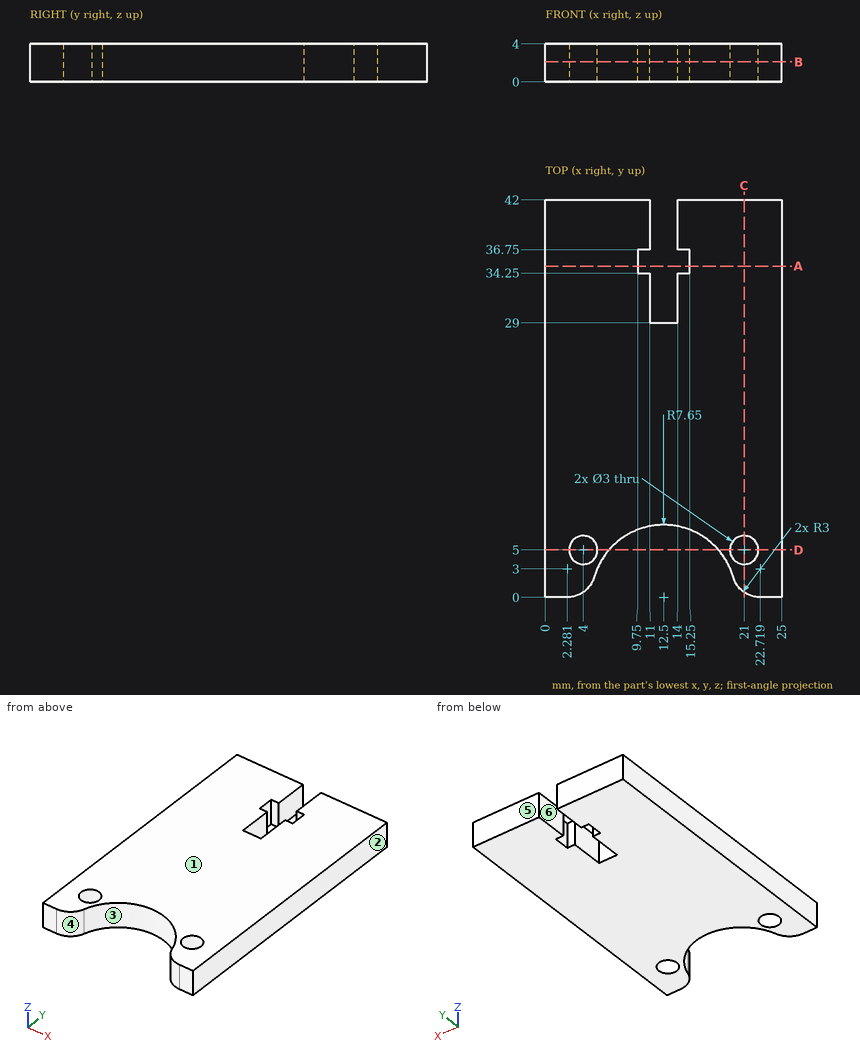
Could you check a few things on this drawing? It's one solid part, dimensions in mm from its lowest x, y, z. A direction names the side the tool comes from. Coordinates: 2 decimals unless noted, no trailing zeros. Order: outer loops, then holes, each group sorted by start corner. A loop starts at its lowest first (then second) coordinate and runs counter-clockwise, first axis right, second up. Notation, with made-up numbers: M 48.25,-21 L 57.25,-21 A23 ccw 57.25,1 Z; hole C -3.5,54 d8. An arc over 180 degrees is marked long. Use a Markdown table: item, result. Add a question column.
Q1. I want a section at A-A on y = 35. List the corners of the cut face in (x, z) for me, then the cut area to 3 significant figures.
Q2. I'm going to push flat-ended pins straight in: pin 1 (1.4 mm diameter, centred on x = 10, z = 2.5, fed in from -Y); pin 2 (1.5 mm diameter, centred on x = 12.5, z = 3, fed in from +Y); pin 3 (1.4 mm diameter, centred on x = 14.5, z = 1.5, fed in from -Y). Where does each tip first touch, or does it pass through?
Q3. We'd pull the mould along X, two halves only. Please class the marked faces 1, 2 and 3: pulls with the +X half, pulls with the -X half, needs draft (parallel to the pull), parting line crosses it, or undercut.
Q4. If I drill on L1, parallel to X at y = 4.5, z = 1.5 (1 decimal); L2, parallel to X at y = 6, z = 0.5 (1 decimal); L3, parallel to X at y = 38, z = 3.75, over which ranges is the centre line in solid material (lowest first)?
Q5. I want a section at B-B on z = 2.1. Give the number of separate pieces and of enclosed holes in the cut face, then the cut area to 3 significant figures.
Q6. Which directions (+Z, -Z, +X, -X, +Y, -Y) give clear straight access to the entire face, cutting with the end or side of a thin tool? Please do the marked faces 4, 5 and 6.
Q7. I want a section at C-C on x = 21. List the corners of the cut face in (y, z) for me.
Q8. I want a section at D-D on y = 5. List the corners of the cut face in (x, z) for me.
Checked values:
| question | item | result |
|---|---|---|
| 1 | outline | M 0,0 L 9.75,0 L 9.75,4 L 0,4 Z; M 15.25,0 L 25,0 L 25,4 L 15.25,4 Z |
| 1 | area | 78.0 mm² |
| 2 | pin 1 | y = 6.95 |
| 2 | pin 2 | y = 29 |
| 2 | pin 3 | y = 7.16 |
| 3 | face 1 | needs draft |
| 3 | face 2 | pulls with the +X half |
| 3 | face 3 | undercut |
| 4 | L1 | 0 to 2.6, 5.4 to 6.3, 18.7 to 19.6, 22.4 to 25 |
| 4 | L2 | 0 to 2.9, 5.1 to 7.8, 17.2 to 19.9, 22.1 to 25 |
| 4 | L3 | 0 to 11, 14 to 25 |
| 5 | separate pieces | 1 |
| 5 | enclosed holes | 2 |
| 5 | area | 896 mm² |
| 6 | face 4 | +Z, -Z, -Y |
| 6 | face 5 | +Z, -Z, +X, -X, +Y |
| 6 | face 6 | +Z, -Z, +Y |
| 7 | outline | M 0.54,0 L 3.5,0 L 3.5,4 L 0.54,4 Z; M 6.5,0 L 42,0 L 42,4 L 6.5,4 Z |
| 8 | outline | M 0,0 L 2.5,0 L 2.5,4 L 0,4 Z; M 5.5,0 L 6.71,0 L 6.71,4 L 5.5,4 Z; M 18.29,0 L 19.5,0 L 19.5,4 L 18.29,4 Z; M 22.5,0 L 25,0 L 25,4 L 22.5,4 Z |
